from build123d import *

# Parameters (mm, degrees)
F1_DEPTH = 50
F2_T     = -4
F4_D     = 22
F4_DEPTH = 4
F4_TIP   = 6.6094668093
F5_R     = 5


# Not quite as in the source:
# - a feature names something its author has since deleted; it is built from what else it names


with BuildPart() as f1:
    # F0 (on Front) → F1 (new body)
    with BuildSketch(Plane.XZ):
        Polygon((250, 50), (-250, 50), (-250, -50), (-150, -50), (250, -50), align=None)
    extrude(amount=F1_DEPTH)

    # F2
    f2_openings = [f1.faces().sort_by_distance(p)[0] for p in [
        (250, -25, 0),
        (-250, -25, 0),
    ]]
    offset(amount=F2_T, openings=f2_openings)

    # F4
    with Locations(Plane(origin=(0, 0, -50), x_dir=(1, 0, 0), z_dir=(0, 0, -1))):
        with Locations((0, 25)):
            Hole(F4_D / 2, depth=F4_DEPTH)
            with Locations((0, 0, -(F4_DEPTH + F4_TIP / 2))):  # 118° drill point
                Cone(0, F4_D / 2, F4_TIP, mode=Mode.SUBTRACT)

    # F5
    f5_edges = [f1.edges().sort_by_distance(p)[0] for p in [
        (0, -50, 50),
        (0, -50, -50),
        (0, 0, -50),
        (0, 0, 50),
        (0, -4, -46),
        (0, -46, -46),
        (0, -46, 46),
        (0, -4, 46),
    ]]
    fillet(f5_edges, radius=F5_R)


solid = f1.part
Can you work these out from the model? Positions are in its coordinate system, mm. A direction names the side the tool comes from. Give positions to 0.01 mm unless a question says otherwise; leave off trailing zeros. Loops run counter-clockwise (first coordinate to the right, second up) from the corner with the lowest first, then second, coordinate; pieces in that order, holes last. Notation, with made-up numbers: (80.25, 19.5) -> (121.25, 19.5) arc R14 cw to (121.25, 44.5) -> close; hole circle Ø4 at (87.5, 63). An arc over 180 degrees is marked (long way). Write item = value, one per line.
1) Suppose I cut it at A-A on y = -25. Write out the boundary of the cut face in (x, z).
Check result:
outline = (-250, -50) -> (-11, -50) -> (-11, -46) -> (-250, -46) -> close; (-250, 46) -> (250, 46) -> (250, 50) -> (-250, 50) -> close; (11, -50) -> (250, -50) -> (250, -46) -> (11, -46) -> close
2) Suppose I cut it at B-B on z = -34.5. Write out the boundary of the cut face in (x, y).
Check result:
outline = (-250, -50) -> (250, -50) -> (250, -46) -> (-250, -46) -> close; (-250, -4) -> (250, -4) -> (250, 0) -> (-250, 0) -> close
3) Thinking about a two-plate mould opening in Z: for faces 4 (the flat face through (-3, -46, 1)), 5 (the flat face through (-3, -11, -50)), 6 (the flat face through (-250, -47, 0)), which applies, released by +Z, released by -Z, zero draft, split by the parting line, or undercut?
Check result:
face_4 = undercut
face_5 = released by -Z
face_6 = zero draft
4) Will this pin go through, and if not, where does the flat tip stop? pin 1 (13 mm diameter, centred on x = 0, y = -25, fed in from -Z).
Check result:
pin_1 = 46
5) I need wall thicknesses on L1, parallel to Z at x = -57.5, y = -38; L2, parallel to Y at x = -150.5, z = 35.5; L3, parallel to Z at x = -85, y = -44. Which ranges of each line are inside material? Lowest first, please. Write a range as from..to.
Check result:
L1 = -50..-46, 46..50
L2 = -50..-46, -4..0
L3 = -50..-45, 45..50
6) Suppose I cut it at D-D on x = 0. Write out the boundary of the cut face in (y, z), then the cut area to 3 significant figures.
Check result:
outline = (-50, -45) arc R5 ccw to (-45, -50) -> (-36, -50) -> (-36, -46) -> (-41, -46) arc R5 cw to (-46, -41) -> (-46, 41) arc R5 cw to (-41, 46) -> (-9, 46) arc R5 cw to (-4, 41) -> (-4, -41) arc R5 cw to (-9, -46) -> (-14, -46) -> (-14, -50) -> (-5, -50) arc R5 ccw to (0, -45) -> (0, 45) arc R5 ccw to (-5, 50) -> (-45, 50) arc R5 ccw to (-50, 45) -> close
area = 1,050 mm2
7) Suppose I cut it at C-C on x = 146. Write out the boundary of the cut face in (y, z).
Check result:
outline = (-50, -45) arc R5 ccw to (-45, -50) -> (-5, -50) arc R5 ccw to (0, -45) -> (0, 45) arc R5 ccw to (-5, 50) -> (-45, 50) arc R5 ccw to (-50, 45) -> close; hole (-46, -41) arc R5 ccw to (-41, -46) -> (-9, -46) arc R5 ccw to (-4, -41) -> (-4, 41) arc R5 ccw to (-9, 46) -> (-41, 46) arc R5 ccw to (-46, 41) -> close
8) For faces 1 (the cylindrical face through (2.38, -14.26, -47.97)), 2 (the flat face through (250, -47, 0)), 3 (the flat face through (3, -25, 46)), which set-ups out of +Z, -Z, +X, -X, +Y, -Y let a thin tool reach every point of the face, with its end or its side?
Check result:
face_1 = -Z
face_2 = +Z, -Z, +X, +Y, -Y
face_3 = +X, -X
